from build123d import *

# Parameters (mm, degrees)
F0_R      = 29.75
F1_DEPTH  = 6
F3_D      = 40
F5_DEPTH  = 6
F7_D      = 40
F9_D      = 7
F10_W     = 10
F10_H     = 65.1724559439
F11_DEPTH = 3
F12_W     = 60
F12_H     = 10
F13_DEPTH = 3


with BuildPart() as f1:
    # F0 (on Top) → F1 (new body)
    with BuildSketch(Plane.XY):
        Circle(F0_R)
    extrude(amount=F1_DEPTH)

    # F3 (through all)
    with Locations(Plane(origin=(0, 0, 0), x_dir=(1, 0, 0), z_dir=(0, 0, -1))):
        with Locations((0, 0)):
            Hole(F3_D / 2)

    # F4 (on face) → F5 (join)
    with BuildSketch(Plane.XY.offset(6)):
        with BuildLine():
            add(Edge.make_bspline(
                [(-51.4080040157, 0), (-48.3840033412, 7.9380003735), (-35.2209347961, 22.8401058322), (-13.735502027, 28.9573147893), (0, 29.75)],
                knots=[0, 0, 0, 0, 0.4596753041, 1, 1, 1, 1], degree=3))
            add(Edge.make_bspline(
                [(-51.4080040157, 0), (-48.3840033412, -7.9380003735), (-35.2209347961, -22.8401058322), (-13.735502027, -28.9573147893), (0, -29.75)],
                knots=[0, 0, 0, 0, 0.4596753041, 1, 1, 1, 1], degree=3))
            add(Edge.make_bspline(
                [(51.4080040157, 0), (48.3840033412, -7.9380003735), (35.2209347961, -22.8401058322), (13.735502027, -28.9573147893), (0, -29.75)],
                knots=[0, 0, 0, 0, 0.4596753041, 1, 1, 1, 1], degree=3))
            add(Edge.make_bspline(
                [(51.4080040157, 0), (48.3840033412, 7.9380003735), (35.2209347961, 22.8401058322), (13.735502027, 28.9573147893), (0, 29.75)],
                knots=[0, 0, 0, 0, 0.4596753041, 1, 1, 1, 1], degree=3))
        make_face()
    extrude(amount=F5_DEPTH)

    # F7 (through all)
    with Locations(Plane.XY.offset(12)):
        with Locations((0, 0)):
            Hole(F7_D / 2)

    # F9 (through all)
    with Locations(Plane.XY.offset(12)):
        with Locations((-41.5, 0), (41.5, 0)):
            Hole(F9_D / 2)

    # F10 (on face) → F11 (cut)
    with BuildSketch(Plane.XY.offset(12)):
        Rectangle(F10_W, F10_H)
    extrude(amount=-F11_DEPTH, mode=Mode.SUBTRACT)

    # F12 (on face) → F13 (cut)
    with BuildSketch(Plane.XY.offset(12)):
        Rectangle(F12_W, F12_H)
    extrude(amount=-F13_DEPTH, mode=Mode.SUBTRACT)


solid = f1.part
Verification items for the finished model (mm, model axes). A direction names the side the tool comes from. Coordinates: 2 decimals unless noted, no trailing zeros. Write each question's results on one line, items separated by ' | '.
1) Gauge pin test, flat ends, axial feed: pin 1 Ø2 at (y, z) = (-10, 5.5) entering from +X; pin 2 Ø8 at (x, y) = (0.5, 25.5) entering from +Z; pin 3 Ø3.5 at (x, z) = (-23.5, 11) entering from +Y. Record the tip position at first contact, or that the pin passes through.
Solved:
pin 1: stops at x = 46.27 | pin 2: stops at z = 9 | pin 3: stops at y = 25.81
2) Scan lines: line 1 along Y through (x, z) = (0, 8.25); line 2 along X through (y, z) = (-10, 9.75); line 3 along X through (y, z) = (-13.5, 8.25). Record each from-to range of solid material in increasing order. Write a range as [from, to].
Solved:
line 1: y = [-29.75, -20], [20, 29.75] | line 2: x = [-45.59, -17.32], [17.32, 45.59] | line 3: x = [-42.42, -14.76], [14.76, 42.42]
3) Access from +Z, -Z, +X, -X, +Y, -Y to the whole of each face (thin tool, end or side, straight path). Record for faces 1 (the face through (-23, 7, 12)), 2 (the face through (5, -24, 11)), 3 (the face through (-33, 0, 6)), 4 (the face through (30, 0, 11)).
Solved:
face 1: +Z, +X, -X, +Y, -Y | face 2: +Z, +Y, -Y | face 3: -Z, -X | face 4: +Z
4) Release check for a two-part mould opening along X. For faces 5 (the face through (15.993, 25.085, 2.958)), 6 (the face through (33, 0, 6)), 7 (the face through (0, -24, 9)) record: pulls with the +X half, pulls with the -X half, needs draft (parallel to the pull), parting line crosses it, or undercut.
Solved:
face 5: parting line crosses it | face 6: needs draft | face 7: undercut
5) Section check A-A on z = 7.25. Give the number of separate pieces and of enclosed holes in the cut face, plus the area to 3 significant figures.
Solved:
separate pieces: 1 | enclosed holes: 3 | area: 3,120 mm²
